```python
from build123d import *

# Parameters (mm, degrees)
SKETCH_1_W            = 150.5
SKETCH_1_H            = 63.5
EXTRUDE_1_DEPTH       = 93.5
SKETCH_2_W            = 1
SKETCH_2_H            = 7
CUT_EXTRUDE_831_DEPTH = 136.783145125


with BuildPart() as part:
    # 草图1 → 拉伸1 (new body)
    with BuildSketch(Plane.XY):
        Rectangle(SKETCH_1_W, SKETCH_1_H)
    extrude(amount=EXTRUDE_1_DEPTH)

    # 扫描1: sweep along a path in 草图3
    with BuildLine(Plane(origin=(0, 19, 0), x_dir=(-1, 0, 0), z_dir=(0, 1, 0))) as sweep_1_path:
        Line((59.75, 0), (59.75, -4))
        Line((59.75, -4), (48.75, -4))
    # 草图2 → 扫描1 (sweep)
    with BuildSketch(Plane(origin=(0, 0, 0), x_dir=(-1, 0, 0), z_dir=(0, 0, -1))):
        with Locations((59.75, 21.25)):
            Rectangle(SKETCH_2_W, SKETCH_2_H)
    sweep_1 = sweep(path=sweep_1_path.line, transition=Transition.RIGHT)

    # 镜向1: 扫描1 across plane
    add(sweep_1.mirror(Plane.ZX))

    # 草图5 → Cut-Extrude 831 (cut, through all)
    with BuildSketch(Plane.XZ.offset(31.75)):
        Polygon((-75.25, 0), (-74.5, 93.5), (-75.25, 93.5), align=None)
        Polygon((74.5, 93.5), (75.25, 93.5), (75.25, 0), align=None)
    extrude(amount=-CUT_EXTRUDE_831_DEPTH, mode=Mode.SUBTRACT)


solid = part.part
```
Model file for the job. Use its own axes, mm. A direction names the side the tool comes from. Give positions to 0.01 mm unless a question says otherwise; leave off trailing zeros. Write each loop counter-clockwise with the first axis right and the second up, starting at its lowest first coordinate (ties: lowest second). Pieces come first, ordered by that corner, then holes. Notation, with made-up numbers: M 30,68 L 38,68 A29 cw 38,88 Z; hole C -34.75,-33.5 d10. An arc over 180 degrees is marked long. Use a Markdown table: item, result.
1) Pin check, flat tips, straight feed: pin 1 (1.1 mm diameter, centred on y = -21, z = -4, fed in from +X); pin 2 (1.4 mm diameter, centred on x = -56, z = -2.5, fed in from -Y); pin 3 (1.5 mm diameter, centred on y = 7.5, z = 55.5, fed in from -X); pin 4 (1 mm diameter, centred on y = 12, z = 42, fed in from +X). Stop position of each tip, or through.
Responses:
| item | result |
|---|---|
| pin 1 | stops at x = -48.75 |
| pin 2 | passes through |
| pin 3 | stops at x = -74.81 |
| pin 4 | stops at x = 74.92 |
2) Cut at C-C (y = -14). List the corners of the cut face in (x, z).
Responses:
| item | result |
|---|---|
| outline | M -75.25,0 L 75.25,0 L 74.5,93.5 L -74.5,93.5 Z |
3) Pull direction Y, two halves, no side cores. Call faces 1 (the flat face through (-1, 31.75, 46)), 2 (the flat face through (-1, -31.75, 46)), 3 (the flat face through (-55, 17.75, -4)), 4 (the flat face through (-54, -21, -4.5)): +Y half, -Y half, draft (parallel to the pull), parting line (faces both ways), or undercut.
Responses:
| item | result |
|---|---|
| face 1 | +Y half |
| face 2 | -Y half |
| face 3 | undercut |
| face 4 | draft |
4) Cut at B-B (x = -28.5). List the corners of the cut face in (y, z).
Responses:
| item | result |
|---|---|
| outline | M -31.75,0 L 31.75,0 L 31.75,93.5 L -31.75,93.5 Z |
5) Tool access for faces 5 (the flat face through (-56, -24.75, -4)), 6 (the flat face through (-56, 24.75, -4)), 7 (the flat face through (-60.25, 21, -2)), 8 (the flat face through (-54, 21, -3.5)), 9 (the flat face through (-55, -17.75, -4)): list every direction of +Z, -Z, +X, -X, +Y, -Y with a clear straight run to the whole face (end or side of a thin tool).
Responses:
| item | result |
|---|---|
| face 5 | -Z, +X, -X, -Y |
| face 6 | -Z, +X, -X, +Y |
| face 7 | -Z, -X, +Y, -Y |
| face 8 | +X, +Y, -Y |
| face 9 | -Z, +X, -X |
6) Cut at A-A (y = 23). List the corners of the cut face in (x, z).
Responses:
| item | result |
|---|---|
| outline | M -75.25,0 L -60.25,0 L -60.25,-4.5 L -48.75,-4.5 L -48.75,-3.5 L -59.25,-3.5 L -59.25,0 L 75.25,0 L 74.5,93.5 L -74.5,93.5 Z |
7) Drill centre lines: line 1 (Z direction, x = -66, y = 8); line 2 (X direction, y = -9, z = 37); line 3 (X direction, y = -22.5, z = 13.5). Where is each one in solid material? Low to high. Write a range as from..to.
Responses:
| item | result |
|---|---|
| line 1 | z = 0..93.5 |
| line 2 | x = -74.95..74.95 |
| line 3 | x = -75.14..75.14 |
